```python
from build123d import *

# Parameters (mm, degrees)
SKETCH_1_W          = 46
SKETCH_1_H          = 100
SKETCH_1_R          = 1.25
SKETCH_1_R_2        = 1.5
EXTRUDE_1_DEPTH     = 2
FILLET_1_R          = 2
SKETCH_2_W          = 10
SKETCH_2_H          = 30
CUT_EXTRUDE_1_DEPTH = 80.429213769
FILLET_2_R          = 3


with BuildPart() as part:
    # 草图1 → 凸台-拉伸1 (new body)
    with BuildSketch(Plane(origin=(0, 0, 0), x_dir=(1, 0, 0), z_dir=(0, 1, 0))):
        with Locations((18, 18)):
            Rectangle(SKETCH_1_W, SKETCH_1_H)
        with Locations(Location((0, 36, 0), (0, 0, 270))):
            Circle(SKETCH_1_R, mode=Mode.SUBTRACT)
        with Locations(Location((36, 36, 0), (0, 0, 270))):
            Circle(SKETCH_1_R, mode=Mode.SUBTRACT)
        with Locations(Location((0, 0, 0), (0, 0, 270))):
            Circle(SKETCH_1_R, mode=Mode.SUBTRACT)
        with Locations(Location((36, 0, 0), (0, 0, 270))):
            Circle(SKETCH_1_R, mode=Mode.SUBTRACT)
        with Locations(Location((0, 63, 0), (0, 0, 270))):
            Circle(SKETCH_1_R_2, mode=Mode.SUBTRACT)
        with Locations(Location((36, 63, 0), (0, 0, 270))):
            Circle(SKETCH_1_R_2, mode=Mode.SUBTRACT)
        with Locations(Location((36, -27, 0), (0, 0, 90))):
            Circle(SKETCH_1_R_2, mode=Mode.SUBTRACT)
        with Locations(Location((0, -27, 0), (0, 0, 90))):
            Circle(SKETCH_1_R_2, mode=Mode.SUBTRACT)
        with Locations(Location((3, 44.83, 0), (0, 0, 270))):
            Circle(SKETCH_1_R_2, mode=Mode.SUBTRACT)
        with Locations(Location((33, 44.83, 0), (0, 0, 270))):
            Circle(SKETCH_1_R_2, mode=Mode.SUBTRACT)
        with Locations(Location((18, 0, 0), (0, 0, 270))):
            Circle(SKETCH_1_R_2, mode=Mode.SUBTRACT)
    extrude(amount=EXTRUDE_1_DEPTH)

    # 圆角1
    fillet_1_edges = [part.edges().sort_by_distance(p)[0] for p in [
        (-5, 1, -68),
        (41, 1, -68),
        (41, 1, 32),
        (-5, 1, 32),
    ]]
    fillet(fillet_1_edges, radius=FILLET_1_R)

    # 草图2 → 切除-拉伸1 (cut, through all)
    with BuildSketch(Plane(origin=(0, 2, 0), x_dir=(1, 0, 0), z_dir=(0, 1, 0))):
        with Locations((0, 18)):
            Rectangle(SKETCH_2_W, SKETCH_2_H)
        with Locations((36, 18)):
            Rectangle(SKETCH_2_W, SKETCH_2_H)
    extrude(amount=-CUT_EXTRUDE_1_DEPTH, mode=Mode.SUBTRACT)

    # 圆角2
    fillet_2_edges = [part.edges().sort_by_distance(p)[0] for p in [
        (-5, 1, -3),
        (-5, 1, -33),
        (41, 1, -33),
        (41, 1, -3),
    ]]
    fillet(fillet_2_edges, radius=FILLET_2_R)


solid = part.part
```
Geometry check sheet. Reference: the model listing, model coordinates, mm. A direction names the side the tool comes from. Round coordinates to 2 decimals unless told otherwise and drop trailing zeros. Loops run counter-clockwise (first coordinate to the right, second up) from the corner with the lowest first, then second, coordinate; pieces in that order, holes last. Notation, with made-up numbers: (89, 37) - (100, 37) arc R5 ccw to (100, 42) - close; hole circle Ø11 at (-11.5, -11.5). An arc over 180 degrees is marked (long way). Write item = value, one per line. Start each with the question number.
1. Section check D-D on z = -23.5. Enter the section's corners in (x, y), then the cut area to 3 significant figures.
2. Section check C-C on y = 0.5. Give the number of separate pieces and of enclosed holes in the cut face, then the cut area to 3 significant figures.
3. Section check A-A on x = 18. Enter the section's corners in (y, z), then the cut area to 3 significant figures.
4. Mould release check, pull along Z, two halves, no side actions. Record for faces 1 (the face through (35.425, 0.986, -61.614)), 2 (the face through (41, 1, -51)): released by +Z, released by -Z, zero draft, split by the parting line, or undercut.
5. Thickness scan on line 1 (X direction, y = 0.4, z = -45); line 2 (X direction, y = 1.8, z = 1); line 3 (X direction, y = 0.65, z = -63). Record the ranges inside material, lowest first.
6. Section check B-B on x = 33. Enter the section's corners in (y, z), then the cut area to 3 significant figures.
7. Set-up check for faces 3 (the face through (1, 1, -33)), 4 (the face through (0.05, 0.99, -37.25)), 5 (the face through (34, 1, -33)): record each of +Z, -Z, +X, -X, +Y, -Y from which the full face is reachable in a straight line by a thin tool's end or side.
Working result:
q1.outline = (5, 0) - (31, 0) - (31, 2) - (5, 2) - close
q1.area = 52.0 mm^2
q2.separate_pieces = 1
q2.enclosed_holes = 11
q2.area = 3,920 mm^2
q3.outline = (0, -68) - (2, -68) - (2, -1.5) - (0, -1.5) - close; (0, 1.5) - (2, 1.5) - (2, 32) - (0, 32) - close
q3.area = 194 mm^2
q4.face_1 = undercut
q4.face_2 = zero draft
q5.line_1 = -5 to 1.51, 4.49 to 31.51, 34.49 to 41
q5.line_2 = -5 to -0.75, 0.75 to 16.88, 19.12 to 35.25, 36.75 to 41
q5.line_3 = -5 to -1.5, 1.5 to 34.5, 37.5 to 41
q6.outline = (0, -68) - (2, -68) - (2, -46.33) - (0, -46.33) - close; (0, -43.33) - (2, -43.33) - (2, -33) - (0, -33) - close; (0, -3) - (2, -3) - (2, 32) - (0, 32) - close
q6.area = 134 mm^2
q7.face_3 = -X, +Y, -Y
q7.face_4 = +Y, -Y
q7.face_5 = +X, +Y, -Y
